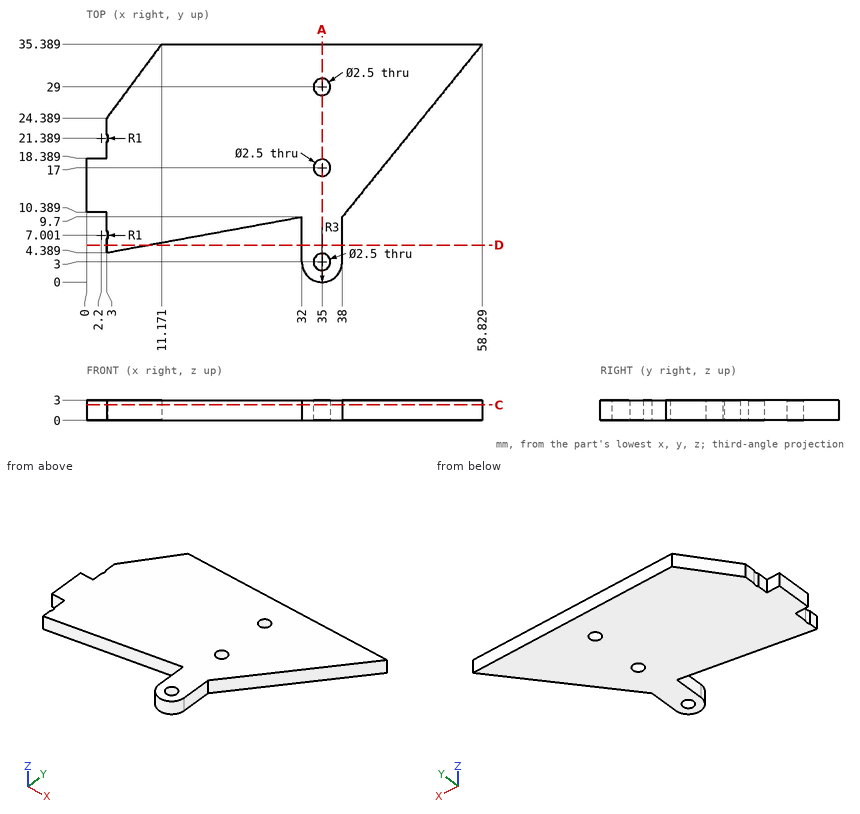
Drawing for the job (mm, zero at the part's lowest x, y, z). Coordinates: 2 decimals unless noted, no trailing zeros. Write each loop counter-clockwise with the first axis right and the second up, starting at its lowest first coordinate (ties: lowest second). Pieces come first, ordered by that corner, then holes. Notation, with made-up numbers: (64, 13.25) - (106, 13.25) arc R17 ccw to (106, 30.25) - close; hole circle Ø2 at (22, -6.75). An arc over 180 degrees is marked (long way). Write each question's results on one line, items separated by ' | '. Start each with the question number.
1) Cut at A-A (x = 35). Write the cut outline in (y, z).
2) Probe line 1 along Y through (x, z) = (35, 1.95); line 2 along X through (y, z) = (18, 2.5); line 3 along X through (y, z) = (4, 2.35). List the from-to ranges inside material, lowest first. Write a range as from..to.
3) Cut at D-D (y = 5.5). Write the cut outline in (x, z).
4) Flat gauge pins, fed straight in: P1, Ø1.5, axis at x = 8.5, y = 4, coming from the -Z side; P2, Ø1.4, axis at y = 9, z = 2, coming from the -X side; P3, Ø0.9, axis at x = 2, z = 1, coming from the +Y side; P4, Ø1.5, axis at x = 1, z = 2, coming from the -Y side. Where does each tip first touch, or does it go through?
5) Cut at C-C (z = 2.3). Write the cut outline in (x, y), then the cut area to 3 significant figures.
Returned:
1) outline: (0, 0) - (1.75, 0) - (1.75, 3) - (0, 3) - close; (4.25, 0) - (15.75, 0) - (15.75, 3) - (4.25, 3) - close; (18.25, 0) - (27.75, 0) - (27.75, 3) - (18.25, 3) - close; (30.25, 0) - (35.39, 0) - (35.39, 3) - (30.25, 3) - close
2) line 1: 0..1.75, 4.25..15.75, 18.25..27.75, 30.25..35.39 | line 2: 0..34.25, 35.75..44.73 | line 3: 32..34.25, 35.75..38
3) outline: (3, 0) - (9.07, 0) - (9.07, 3) - (3, 3) - close; (32, 0) - (38, 0) - (38, 3) - (32, 3) - close
4) P1: through | P2: x = 3 | P3: y = 18.39 | P4: y = 10.39
5) outline: (0, 10.39) - (3, 10.39) - (3, 7.6) arc R1 cw to (3, 6.4) - (3, 4.39) - (32, 9.7) - (32, 3) arc R3 ccw to (38, 3) - (38, 9.7) - (58.83, 35.39) - (11.17, 35.39) - (3, 24.39) - (3, 21.99) arc R1 cw to (3, 20.79) - (3, 18.39) - (0, 18.39) - close; hole circle Ø2.5 at (35, 3); hole circle Ø2.5 at (35, 17); hole circle Ø2.5 at (35, 29) | area: 1,260 mm^2
